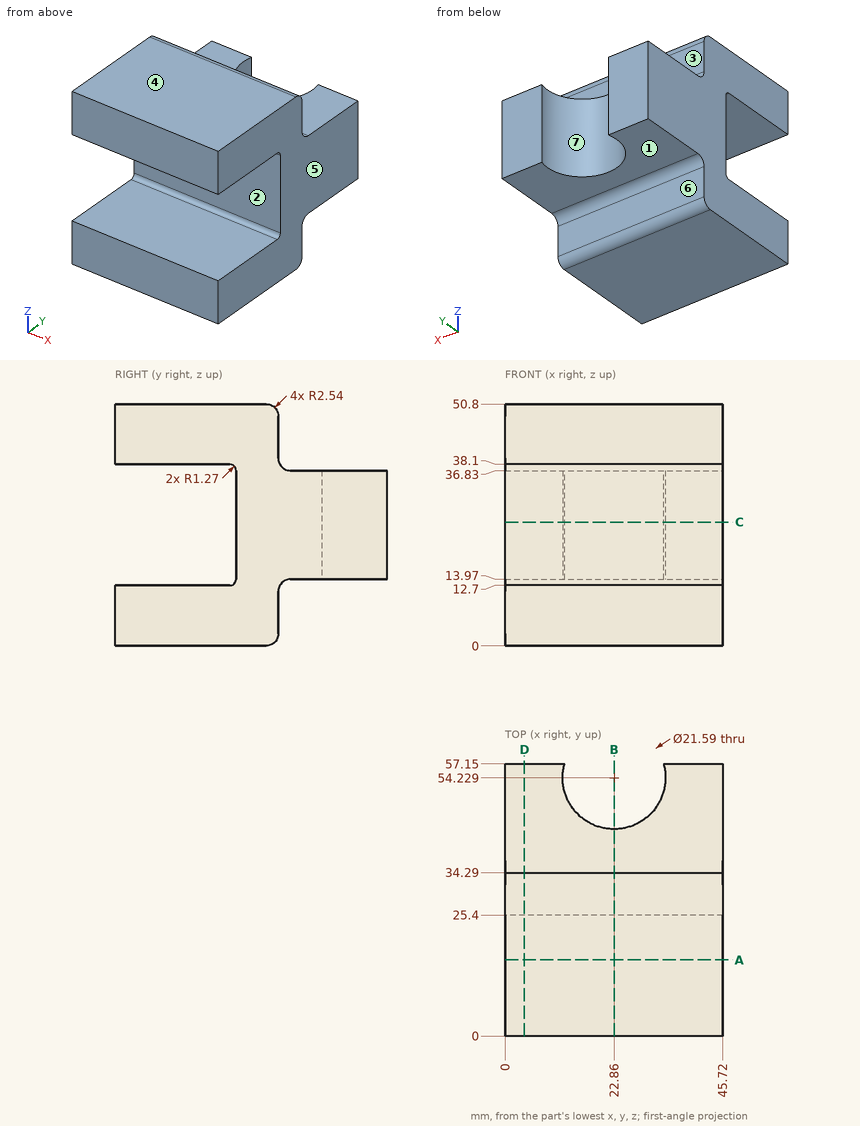
Verification items for this drawing (mm, ordinates from the low corner). A direction names the side the tool comes from. Round coordinates to 2 decimals unless told otherwise and drop trailing zeros. Loops run counter-clockwise (first coordinate to the right, second up) from the corner with the lowest first, then second, coordinate; pieces in that order, holes last. Notation, with made-up numbers: M 1.5,-28 L 6.5,-28 A27 cw 6.5,-10 Z; hole C 24,71.5 d6. An arc over 180 degrees is marked long. Answer as a JSON object with one key per item and string values.
1. Mould release check, pull along Y, two halves, no side actions. Record for the marked faces 5, 6 and 7: pulls with the +Y half, pulls with the -Y half, needs draft (parallel to the pull), parting line crosses it, or undercut.
Reply:
{"face 5": "needs draft", "face 6": "pulls with the +Y half", "face 7": "undercut"}
2. Section check A-A (y = 16). Record the boundary of the cut face in (x, z).
Reply:
{"outline": "M 0,0 L 45.72,0 L 45.72,12.7 L 0,12.7 Z; M 0,38.1 L 45.72,38.1 L 45.72,50.8 L 0,50.8 Z"}
3. Section check D-D (x = 4). Record the boundary of the cut face in (y, z), plus the area to 3 significant figures.
Reply:
{"outline": "M 0,0 L 31.75,0 A2.54 ccw 34.29,2.54 L 34.29,11.43 A2.54 cw 36.83,13.97 L 57.15,13.97 L 57.15,36.83 L 36.83,36.83 A2.54 cw 34.29,39.37 L 34.29,48.26 A2.54 ccw 31.75,50.8 L 0,50.8 L 0,38.1 L 24.13,38.1 A1.27 cw 25.4,36.83 L 25.4,13.97 A1.27 cw 24.13,12.7 L 0,12.7 Z", "area": "1,620 mm²"}
4. Access from +Z, -Z, +X, -X, +Y, -Y to the whole of each face (thin tool, end or side, straight path). Record for the marked faces 1, 2, 3 and 4.
Reply:
{"face 1": "-Z, +X, -X, +Y", "face 2": "+X, -X, -Y", "face 3": "+Z, +X, -X, +Y", "face 4": "+Z, +X, -X, +Y, -Y"}
5. Scan lines: line 1 (Z direction, x = 20.5, y = 10.5); line 2 (X direction, y = 54, z = 18); line 3 (Y direction, x = 22.86, z = 26). Record each from-to range of solid material in increasing order.
Reply:
{"line 1": "z = 0 to 12.7, 38.1 to 50.8", "line 2": "x = 0 to 12.07, 33.65 to 45.72", "line 3": "y = 25.4 to 43.43"}
6. Section check B-B (x = 22.86). Record the boundary of the cut face in (y, z), plus the area to 3 significant figures.
Reply:
{"outline": "M 0,0 L 31.75,0 A2.54 ccw 34.29,2.54 L 34.29,11.43 A2.54 cw 36.83,13.97 L 43.43,13.97 L 43.43,36.83 L 36.83,36.83 A2.54 cw 34.29,39.37 L 34.29,48.26 A2.54 ccw 31.75,50.8 L 0,50.8 L 0,38.1 L 24.13,38.1 A1.27 cw 25.4,36.83 L 25.4,13.97 A1.27 cw 24.13,12.7 L 0,12.7 Z", "area": "1,310 mm²"}
7. Section check C-C (z = 26). Record the boundary of the cut face in (x, y) (3 decimals).
Reply:
{"outline": "M 0,25.4 L 45.72,25.4 L 45.72,57.15 L 33.252,57.15 A10.795 cw long 12.468,57.15 L 0,57.15 Z"}
8. Gauge pin test, flat ends, axial feed: P1, Ø5, axis at x = 22.5, y = 45, coming from the -Z side; P2, Ø1, axis at y = 28.5, z = 43, coming from the -X side; P3, Ø8, axis at x = 23.5, y = 39.5, coming from the -Z side; P4, Ø1.5, axis at x = 6, z = 15, coming from the -Y side. Record the tip position at first contact, or that the pin passes through.
Reply:
{"P1": "stops at z = 13.97", "P2": "stops at x = 0", "P3": "stops at z = 13.59", "P4": "stops at y = 25.4"}
